Autodesk Inventor part; units mm, degrees
ref_plane "YZ Plane" through (0, 0, 0) normal (1, 0, 0) x (0, 1, 0)
ref_plane "XZ Plane" through (0, 0, 0) normal (0, 1, 0) x (-1, 0, 0)
ref_plane "XY Plane" through (0, 0, 0) normal (0, 0, 1) x (1, 0, 0)
sketch "Sketch1" plane through (0, 0, 0) normal (0, 0, 1) x (1, 0, 0)
  circle A0 centre (0, 0) radius 6
  dimension "d0" = 12
extrude "Extrusion1" add sketch "Sketch1" along normal blind 9.5
ref_plane "Work Plane1" through (0, 0, 9) normal (0, 0, 1) x (1, 0, 0)
sketch "Sketch2" plane through (0, 0, 9) normal (0, 0, 1) x (1, 0, 0)
  circle A0 centre (0, 0) radius 6
  circle A1 centre (0, 0) radius 4.25
  dimension "d4" = 8.5
extrude "Extrusion2" cut sketch "Sketch2" against normal blind 1 contours A1
sketch "Sketch3" plane through (0, 0, 9.5) normal (0, 0, 1) x (1, 0, 0)
  circle A0 centre (0, 0) radius 6
  circle A1 centre (0, 0) radius 1.1
  dimension "d7" = 2.2
extrude "Extrusion3" cut sketch "Sketch3" against normal blind 0.5 contours A1
sketch "Sketch4" plane through (0, 0, 0) normal (0, 0, -1) x (-1, 0, 0)
  circle A0 centre (0, 0) radius 6
  circle A1 centre (0, 0) radius 5.25
  dimension "d10" = 10.5
extrude "Extrusion4" cut sketch "Sketch4" against normal blind 0.5 contours A1
fillet "Fillet1" radius 0.5 1 edges at (-6, 0, 9.5)
sketch "Sketch5" plane through (0, 0, 0) normal (0, 0, -1) x (-1, 0, 0)
  circle A0 centre (0, 0) radius 5.25
  circle A1 centre (0, 0) radius 6
  line L0 (2.5416, 4.5938) -> (2.9047, 5.25)
  line L1 (-2.5416, 4.5938) -> (-2.9047, 5.25)
extrude "Extrusion5" cut sketch "Sketch5" against normal blind 0.5 contours A0 L1 A1 L0 picked at (0.1766, 5.7207)
pattern_circular "Circular Pattern1" count 3 over 360 about axis through (0, 0, 0) along (0, 0, 1) of "Extrusion5"
sketch "Sketch6" plane through (0, 0, 0.5) normal (0, 0, -1) x (-1, 0, 0)
  arc A0 (-5.999, -0.1094) -> (-3.0943, -5.1406) centre (0, 0) ccw
  circle A1 centre (0, 3.8) radius 0.3
  dimension "d19" = 0.6
  dimension "d20" = 3.8
extrude "Extrusion6" add sketch "Sketch6" along normal blind 6
sketch "Sketch7" plane through (0, 0, 0.5) normal (0, 0, -1) x (-1, 0, 0)
  arc A0 (-2.5416, 4.5938) -> (-5.2491, -0.0957) centre (0, 0) ccw
  circle A1 centre (0, -3.8) radius 0.3
  dimension "d23" = 0.6
  dimension "d24" = 3.8
extrude "Extrusion7" add sketch "Sketch7" along normal blind 4
chamfer "Chamfer1" distance 0.2 angle 45 2 edges at (0.3, 3.8, -5.5) (0.3, -3.8, -3.5)
sketch "Sketch8" plane through (0, 0, 9.5) normal (0, 0, 1) x (1, 0, 0)
  line L0 (-0.7574, 4.5872) -> (0.6588, 4.5872) construction
  line L1 (0.6588, 4.5872) -> (0.6588, 3.3036) construction
  line L2 (0.6588, 3.3036) -> (-0.7574, 3.3036) construction
  line L3 (-0.7574, 3.3036) -> (-0.7574, 4.5872) construction
  line L4 (0.5858, 3.9175) -> (0.0777, 3.9175)
  line L5 (0.0777, 3.9175) -> (0.0777, 3.4094)
  line L6 (0.0777, 3.4094) -> (-0.09, 3.4094)
  line L7 (-0.09, 3.4094) -> (-0.09, 3.9175)
  line L8 (-0.09, 3.9175) -> (-0.5981, 3.9175)
  line L9 (-0.5981, 3.9175) -> (-0.5981, 4.0791)
  line L10 (-0.5981, 4.0791) -> (-0.09, 4.0791)
  line L11 (-0.09, 4.0791) -> (-0.09, 4.5872)
  line L12 (-0.09, 4.5872) -> (0.0777, 4.5872)
  line L13 (0.0777, 4.5872) -> (0.0777, 4.0791)
  line L14 (0.0777, 4.0791) -> (0.5858, 4.0791)
  line L15 (0.5858, 4.0791) -> (0.5858, 3.9175)
extrude "Extrusion8" cut sketch "Sketch8" against normal blind 0.1
sketch "Sketch9" plane through (0, 0, 9.5) normal (0, 0, 1) x (1, 0, 0)
  circle A0 centre (0, 3.9983) radius 0.824
  circle A1 centre (0, 3.9983) radius 0.8972
extrude "Extrusion9" cut sketch "Sketch9" against normal blind 0.01
ref_plane "Work Plane2" through (0, 0, 3.5) normal (0, 0, 1) x (1, 0, 0)
sketch "Sketch10" plane through (0, 0, 3.5) normal (0, 0, 1) x (1, 0, 0)
  circle A0 centre (0, 0) radius 6
  circle A1 centre (0, 0) radius 5.75
  dimension "d35" = 11.5
extrude "Extrusion10" cut sketch "Sketch10" along normal mid plane 0.1
properties part number "buzzer"
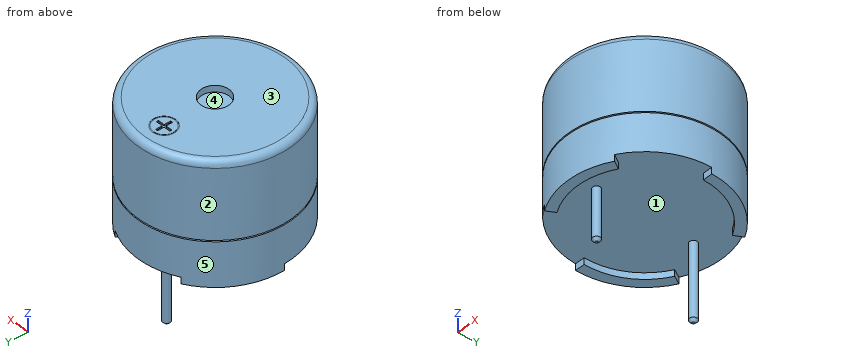
Can you work these out from the model? Positions are in its coordinate system, mm. Face numbers are marked on the shaded views. A direction names the side the tool comes from. Round coordinates to 2 decimals unless told otherwise and drop trailing zeros. Loops run counter-clockwise (first coordinate to the right, second up) from the corner with the lowest first, then second, coordinate; pieces in that order, holes last. Notation, with made-up numbers: M 59,83 L 118,83 A17 cw 118,92 Z; hole C 86,29.5 d7. An arc over 180 degrees is marked long. Answer in a Markdown table with one row per item.
1. Thinking about a two-plate mould opening in Y: for the marked faces 3, 4 and 5, which applies, pulls with the +Y half, pulls with the -Y half, needs draft (parallel to the pull), parting line crosses it, or undercut?
Established:
| item | result |
|---|---|
| face 3 | needs draft |
| face 4 | undercut |
| face 5 | parting line crosses it |
2. On a 3-axis mill with a long thin cutter (end or side, diameter ignored), from which of +Z, -Z, +X, -X, +Y, -Y can I reach the whole of each face in a straight line? I mean the marked faces 1 and 2. Say none if no direction works.
Established:
| item | result |
|---|---|
| face 1 | -Z |
| face 2 | +Z, -Z |
3. If we section it at C-C, the plane z = -4: Please give me the cut outline in (x, y), plus the area to 3 significant figures.
Established:
| item | result |
|---|---|
| outline | C 0,3.8 d0.6 |
| area | 0.283 mm² |
4. Please list where these lines run through material, in increasing order: line 1 (Y direction, x = 0, z = 8.85); line 2 (Z direction, x = 1.5, y = 1); line 3 (Z direction, x = -2.75, y = -3.75). Write a range as from..to.
Established:
| item | result |
|---|---|
| line 1 | -6..-4.25, 4.25..6 |
| line 2 | 0.5..8, 9..9.5 |
| line 3 | 0.5..9.5 |
5. I'm going to push flat-ended pins straight in: pin 1 Ø3 at (x, z) = (4, 1) entering from +Y; pin 2 Ø5.5 at (x, y) = (0, 0.5) entering from -Z; pin 3 Ø5 at (y, z) = (3, 3) entering from +X. Where does each tip first touch, or does it pass through?
Established:
| item | result |
|---|---|
| pin 1 | y = 5.45 |
| pin 2 | z = 0.5 |
| pin 3 | x = 5.98 |
6. If we section it at A-A, the plane z = -2: Please give me the cut outline in (x, y), plus the area to 3 significant figures.
Established:
| item | result |
|---|---|
| outline | C 0,-3.8 d0.6; C 0,3.8 d0.6 |
| area | 0.565 mm² |
7. If we section it at B-B, the plane z = 8.25: Please give me the cut outline in (x, y), plus the area to 3 significant figures.
Established:
| item | result |
|---|---|
| outline | C 0,0 d12; hole C 0,0 d8.5 |
| area | 56.4 mm² |
